Geometry: see drawing. Coordinates: mm, zero at the bounding-box minimum. Coordinates: 2 decimals unless noted, no trailing zeros. Order: outer loops, then holes, each group sorted by start corner. A loop starts at its lowest first (then second) coordinate and runs counter-clockwise, first axis right, second up.
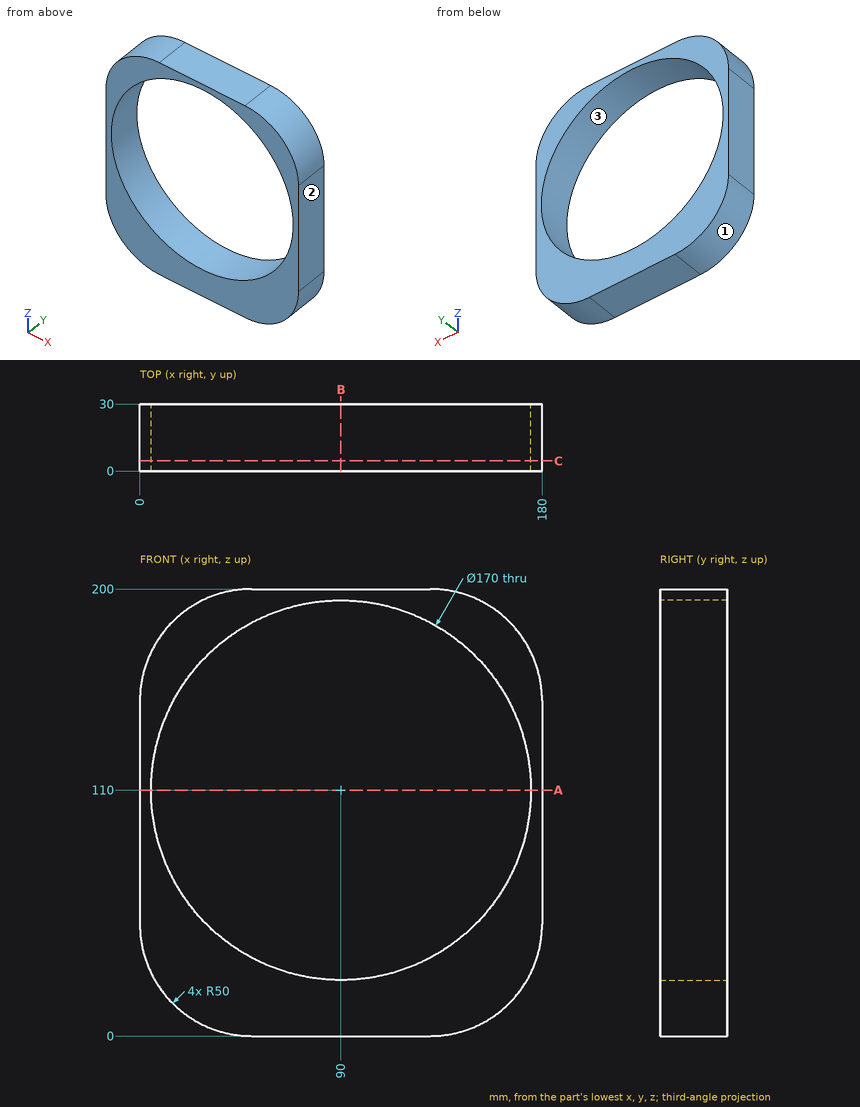
Q1. Material intervals for line 1 along X through (y, z) = (19.75, 110); line 2 along Z through (x, y) = (121.5, 25.75); line 3 along X through (y, z) = (7.25, 122), sorted ascending.
Solutions:
line 1: x = 0 to 5, 175 to 180
line 2: z = 0 to 31.05, 188.95 to 200
line 3: x = 0 to 5.85, 174.15 to 180
Q2. Section query A-A on z = 110. Output: boundary loops of the cut face in (x, y).
Solutions:
outline: (0, 0) - (5, 0) - (5, 30) - (0, 30) - close; (175, 0) - (180, 0) - (180, 30) - (175, 30) - close
Q3. Pin query (flat end, axial travel): P1, Ø1, axis at y = 12.5, z = 47.5, coming from the -X side; P2, Ø5, axis at x = 150.5, y = 10, coming from the +Z side; P3, Ø1, axis at y = 10, z = 40.5, coming from the -X side. Return the tip coordinate at first contact, or that it passes through.
Solutions:
P1: stops at x = 0.04
P2: stops at z = 196.65
P3: stops at x = 0.82
Q4. Section query C-C on y = 4.5. Output: boundary loops of the cut face in (x, z).
Solutions:
outline: (0, 50) arc R50 ccw to (50, 0) - (130, 0) arc R50 ccw to (180, 50) - (180, 150) arc R50 ccw to (130, 200) - (50, 200) arc R50 ccw to (0, 150) - close; hole circle Ø170 at (90, 110)
Q5. Section query B-B on x = 90. Output: boundary loops of the cut face in (y, z).
Solutions:
outline: (0, 0) - (30, 0) - (30, 25) - (0, 25) - close; (0, 195) - (30, 195) - (30, 200) - (0, 200) - close
Q6. Pull-direction query (X, two-part tool) for the marked faces 1, 2 and 3; classes: pulls with the +X half, pulls with the -X half, needs draft (parallel to the pull), parting line crosses it, or undercut.
Solutions:
face 1: pulls with the -X half
face 2: pulls with the +X half
face 3: undercut
